Read the model definition and answer for the solid it produces. Units are mm, in the model's axes. Face numbers are marked on the shaded views. Give positions to 0.01 mm unless a question says otherwise; leave off trailing zeros. Loops run counter-clockwise (first coordinate to the right, second up) from the corner with the lowest first, then second, coordinate; pieces in that order, holes last. Notation, with made-up numbers: (52.5, 78.5) -> (76.5, 78.5) arc R7 ccw to (76.5, 88.5) -> close; hole circle Ø9 at (-3, 33.25). An arc over 180 degrees is marked (long way). One line per item, written item: value. Start each with the question number.
Autodesk Inventor part; units mm, degrees
ref_plane "YZ Plane" through (0, 0, 0) normal (1, 0, 0) x (0, 1, 0)
ref_plane "XZ Plane" through (0, 0, 0) normal (0, 1, 0) x (-1, 0, 0)
ref_plane "XY Plane" through (0, 0, 0) normal (0, 0, 1) x (1, 0, 0)
sketch "Sketch1" plane through (0, 0, 0) normal (0, 0, 1) x (1, 0, 0)
  circle A0 centre (0, 0) radius 34.925
  circle A1 centre (0, 0) radius 9.525
  point P0 (0, 25.4)
  point P1 (0, -25.4)
  point P2 (-26.797, -17.4625)
  point P3 (-26.797, 17.4625)
  point P4 (26.797, 17.4625)
  point P5 (26.797, -17.4625)
  dimension "d0" = 69.85
  dimension "d1" = 19.05
  dimension "d2" = 25.4
  dimension "d3" = 25.4
  dimension "d4" = 26.797
  dimension "d5" = 17.4625
  dimension "d6" = 17.4625
  dimension "d7" = 26.797
extrude "Extrusion1" add sketch "Sketch1" against normal blind 6.35
hole "Hole1" at (-26.797, -17.4625, 0) at (-26.797, 17.4625, 0) at (26.797, 17.4625, 0) at (26.797, -17.4625, 0) direction (0, 0, -1) diameter 2.6416 end through all
hole "Hole2" at (0, 25.4, 0) at (0, -25.4, 0) direction (0, 0, -1) diameter 4.826 end through all countersink diameter 9.525 countersink angle 82
properties part number "Dewalt Drill Drive CIMmotor Adaptor"
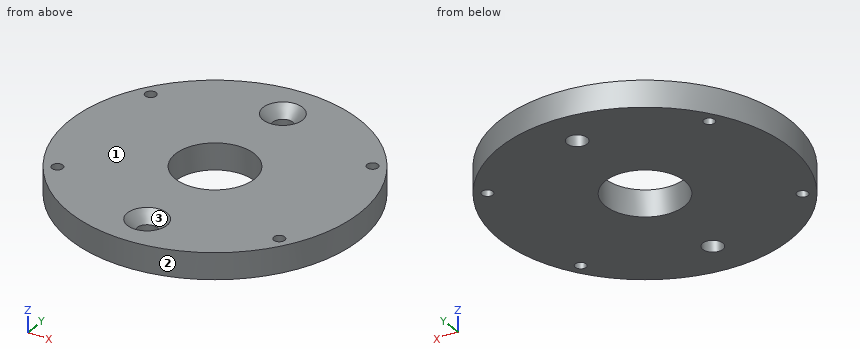
Item 1: Section A-A, the plane y = 0 is taken. Determine the outline of the cut face in (x, z) (3 decimals).
Item 2: Determine the mould class of the marked faces 1, 2 and 3 for opening direction X: pulls with the +X half, pulls with the -X half, needs draft (parallel to the pull), parting line crosses it, or undercut.
Item 3: Section B-B, the plane x = 0 is taken. State how many separate pieces and enclosed holes the cut face has, plus the area to 3 significant figures.
Item 4: Flat-ended cylindrical pins translate along their axes: pin 1 (1.5 mm diameter, centred on y = 16.5, z = -1, fed in from +X); pin 2 (3 mm diameter, centred on x = 24.5, z = -4.5, fed in from -Y); pin 3 (2 mm diameter, centred on x = -26.8, y = -17.46, fed in from -Z); pin 4 (3.5 mm diameter, centred on x = -26.8, y = 17.46, fed in from -Z). Find the tip coordinate at first contact, or state that the pin passes through.
Item 5: Consider L1, parallel to Y at x = 0, z = -3.85 (3 decimals); L2, parallel to X at y = 18, z = -2; L3, parallel to Y at x = 26, z = -4.25. Determine where each line is inside the solid, lowest interval first. Write a range as [from, to].
Item 6: Section D-D, the plane y = -25.4 is taken. Determine the outline of the cut face in (x, z), plus the area to 3 significant figures.
Computed values:
1. outline: (-34.925, -6.35) -> (-9.525, -6.35) -> (-9.525, 0) -> (-34.925, 0) -> close; (9.525, -6.35) -> (34.925, -6.35) -> (34.925, 0) -> (9.525, 0) -> close
2. face 1: needs draft
2. face 2: parting line crosses it
2. face 3: undercut
3. separate pieces: 4
3. enclosed holes: 0
3. area: 249 mm²
4. pin 1: x = 31.17
4. pin 2: y = -26.28
4. pin 3: through
4. pin 4: z = -6.35
5. L1: [-34.925, -27.813], [-22.987, -9.525], [9.525, 22.987], [27.813, 34.925]
5. L2: [-29.93, -28], [-25.59, 25.59], [28, 29.93]
5. L3: [-23.32, -18.52], [-16.41, 16.41], [18.52, 23.32]
6. outline: (-23.97, -6.35) -> (-2.41, -6.35) -> (-2.41, -2.7) -> (-4.76, 0) -> (-23.97, 0) -> close; (2.41, -6.35) -> (23.97, -6.35) -> (23.97, 0) -> (4.76, 0) -> (2.41, -2.7) -> close
6. area: 267 mm²
